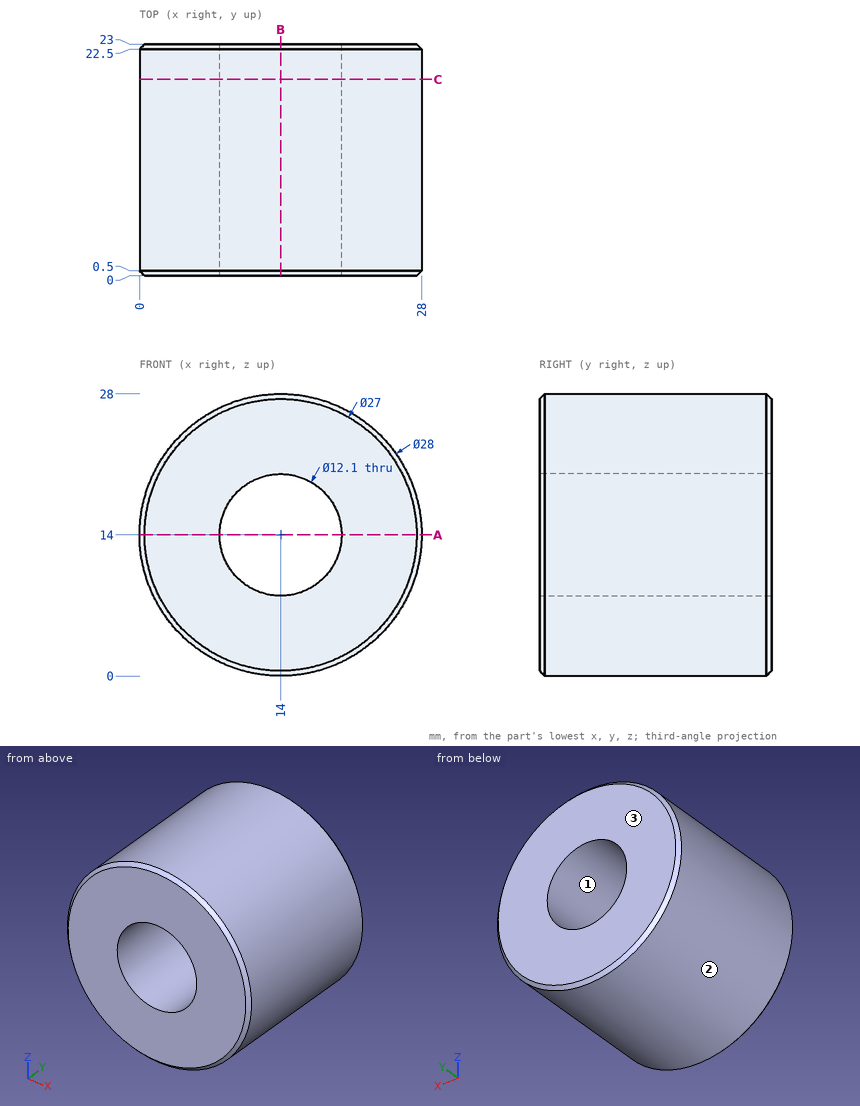
Source: three-view drawing plus pictorial views. Frame: mm from the lowest corner of the part. Give positions to 0.01 mm unless a question says otherwise; leave off trailing zeros. Order: outer loops, then holes, each group sorted by start corner. A loop starts at its lowest first (then second) coordinate and runs counter-clockwise, first axis right, second up.
1. Section C-C on y = 19.5. Return the cut outline in (x, z).
Derived:
outline: circle Ø28 at (14, 14); hole circle Ø12.1 at (14, 14)
2. Mould query, pull axis Z, two halves, no side actions, for the marked faces 1, 2 and 3. Classes: released by +Z, released by -Z, zero draft, split by the parting line, or undercut.
Derived:
face 1: undercut
face 2: split by the parting line
face 3: zero draft
3. Section A-A on z = 14. Return the cut outline in (x, y), and give its area (3 significant figures).
Derived:
outline: (0, 0.5) - (0.5, 0) - (7.95, 0) - (7.95, 23) - (0.5, 23) - (0, 22.5) - close; (20.05, 0) - (27.5, 0) - (28, 0.5) - (28, 22.5) - (27.5, 23) - (20.05, 23) - close
area: 365 mm2
4. Section B-B on x = 14. Return the cut outline in (y, z).
Derived:
outline: (0, 0.5) - (0.5, 0) - (22.5, 0) - (23, 0.5) - (23, 7.95) - (0, 7.95) - close; (0, 20.05) - (23, 20.05) - (23, 27.5) - (22.5, 28) - (0.5, 28) - (0, 27.5) - close
5. Pin query (flat end, axial travel): pin 1 (10 mm diameter, centred on x = 24, y = 8, fed in from +Z); pin 2 (6 mm diameter, centred on y = 6.5, z = 4.5, fed in from -X); pin 3 (6 mm diameter, centred on y = 5.5, z = 7.5, fed in from -X). Return the tip coordinate at first contact, or that it passes through.
Derived:
pin 1: stops at z = 27.08
pin 2: stops at x = 1.6
pin 3: stops at x = 0.44
6. Material intervals for L1, parallel to X at y = 10, z = 14; L2, parallel to Z at x = 14.25, y = 6.25; L3, parallel to X at y = 16.5, z = 8.75, sorted ascending.
Derived:
L1: x = 0 to 7.95, 20.05 to 28
L2: z = 0 to 7.96, 20.04 to 28
L3: x = 1.02 to 10.99, 17.01 to 26.98
